Part print with two shaded views. Sizes in mm from the minimum x, y, z corner. A direction names the side the tool comes from. Round coordinates to 2 decimals unless told otherwise and drop trailing zeros. Write each loop counter-clockwise with the first axis right and the second up, starting at its lowest first coordinate (ties: lowest second). Pieces come first, ordered by that corner, then holes. Notation, with made-up numbers: (25, -25) -> (35, -25) arc R27 cw to (35, 4) -> close; hole circle Ø6 at (-22.75, 4). An arc over 180 degrees is marked (long way). Put each result on its own line as item: value. Start each with the question number.
1. Pull direction Y, two halves, no side cores. Call the marked faces 5, 6 and 7: pulls with the +Y half, pulls with the -Y half, needs draft (parallel to the pull), parting line crosses it, or undercut.
2. Saw through at D-D on z = 7.75. List the corners of the cut face in (x, y) (1 decimal), and give its area (3 significant figures).
3. Saw through at A-A on z = 3. List the corners of the cut face in (x, y).
4. Flat gauge pins, fed straight in: P1, Ø1, axis at y = 24, z = 4.5, coming from the +X side; P2, Ø2, axis at y = 24.5, z = 5.5, coming from the -X side; P3, Ø1.8, axis at x = 12.5, z = 5.5, coming from the -Y side; P4, Ø2, axis at x = 19, z = 4.5, coming from the +Y side. Where does each tip first touch, or does it go through?
5. Saw through at B-B on y = 12. List the corners of the cut face in (x, z).
6. 3-axis set-ups, long thin cutter, end or side, ignore diameter. For the marked faces 1, 2, 3 and 4: which of +Z, -Z, +X, -X, +Y, -Y reach the whole face in a straight line?
7. Saw through at C-C on x = 11.5. List the corners of the cut face in (y, z) (1 decimal).
8. Drill centre lines: line 1 (Y direction, x = 9, z = 6.5); line 2 (Y direction, x = 10.75, z = 7.25) (1 decimal); line 3 (X direction, y = 26.5, z = 6.5). Where is each one in solid material? Low to high. Write a range as from..to.
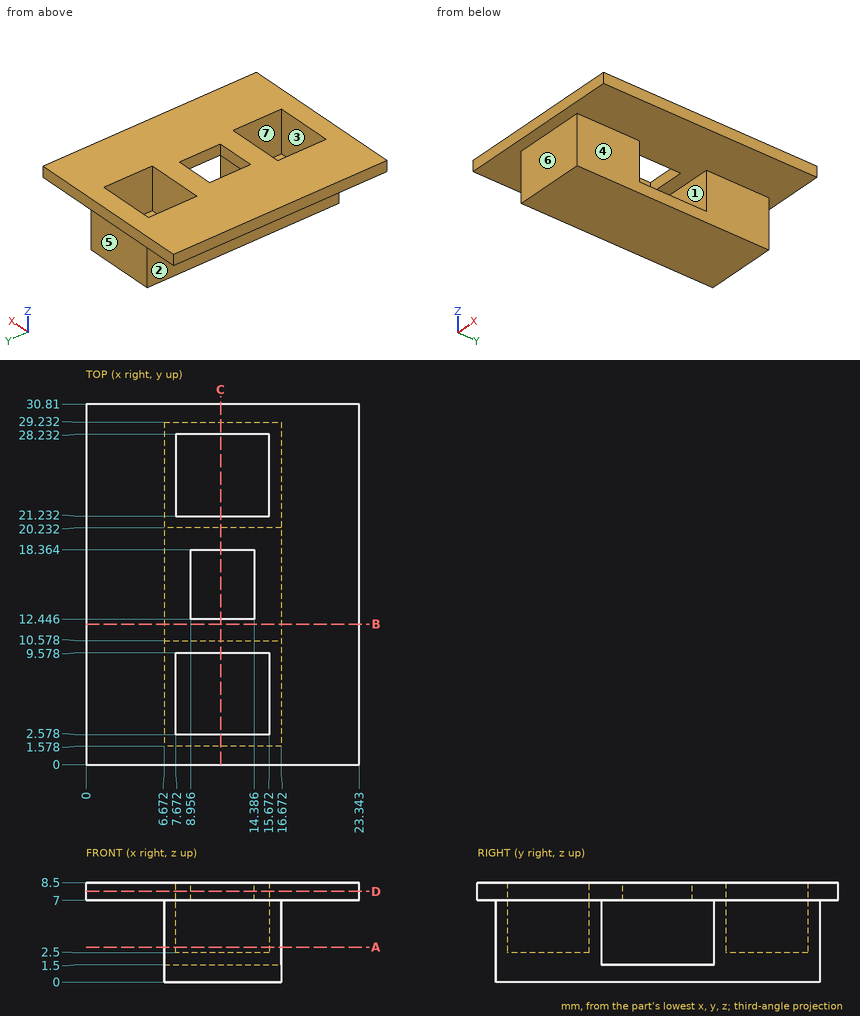
Return value:
1. face 5: pulls with the +Y half
1. face 6: pulls with the -Y half
1. face 7: undercut
2. outline: (0, 0) -> (23.3, 0) -> (23.3, 30.8) -> (0, 30.8) -> close; hole (7.7, 2.6) -> (15.7, 2.6) -> (15.7, 9.6) -> (7.7, 9.6) -> close; hole (7.7, 21.2) -> (15.7, 21.2) -> (15.7, 28.2) -> (7.7, 28.2) -> close; hole (9, 12.4) -> (14.4, 12.4) -> (14.4, 18.4) -> (9, 18.4) -> close
2. area: 575 mm^2
3. outline: (6.67, 1.58) -> (16.67, 1.58) -> (16.67, 10.58) -> (6.67, 10.58) -> close; (6.67, 20.23) -> (16.67, 20.23) -> (16.67, 29.23) -> (6.67, 29.23) -> close; hole (7.67, 2.58) -> (15.67, 2.58) -> (15.67, 9.58) -> (7.67, 9.58) -> close; hole (7.67, 21.23) -> (15.67, 21.23) -> (15.67, 28.23) -> (7.67, 28.23) -> close
4. P1: stops at x = 16.67
4. P2: stops at x = 6.67
4. P3: stops at y = 1.58
4. P4: passes through
5. outline: (0, 7) -> (23.34, 7) -> (23.34, 8.5) -> (0, 8.5) -> close; (6.67, 0) -> (16.67, 0) -> (16.67, 1.5) -> (6.67, 1.5) -> close
6. face 1: +X, -X
6. face 2: -Z, -X, +Y, -Y
6. face 3: +Z
6. face 4: -Z, +X, +Y, -Y
7. outline: (0, 7) -> (1.6, 7) -> (1.6, 0) -> (29.2, 0) -> (29.2, 7) -> (30.8, 7) -> (30.8, 8.5) -> (28.2, 8.5) -> (28.2, 2.5) -> (21.2, 2.5) -> (21.2, 8.5) -> (18.4, 8.5) -> (18.4, 7) -> (20.2, 7) -> (20.2, 1.5) -> (10.6, 1.5) -> (10.6, 7) -> (12.4, 7) -> (12.4, 8.5) -> (9.6, 8.5) -> (9.6, 2.5) -> (2.6, 2.5) -> (2.6, 8.5) -> (0, 8.5) -> close
8. line 1: y = 1.58..2.58, 9.58..10.58, 20.23..21.23, 28.23..29.23
8. line 2: y = 0..2.6, 9.6..12.4, 18.4..21.2, 28.2..30.8
8. line 3: x = 6.67..7.67, 15.67..16.67
